Could you check a few things on this model? Use its own coordinates, in mm. Give positions to 0.01 mm unless a question says otherwise; leave off trailing zeros. Loops run counter-clockwise (first coordinate to the right, second up) from the corner with the lowest first, then second, coordinate; pieces in that order, holes last. Notation, with made-up numbers: M -20.75,69.25 L -5.75,69.25 A15 ccw -5.75,87.25 Z; hole C 38,65 d9. An arc over 180 degrees is marked long. Answer in a Markdown table with one row per item. Add a question column.
1. I'm going to push a flat-ended pin straight in: pin 1 Ø2 at (x, z) = (17.5, -1) entering from +Y. Where does the tip first touch, or does it pass through?
2. If we section it at B-B on x = 24: List the corners of the cut face in (y, z) for me.
3. If we section it at A-A on z = 0: List the corners of the cut face in (x, y) for me.
4. I need wall thicknesses on line 1 along X through (y, z) = (0, 2.15); line 2 along X through (y, z) = (0, 1.75); line 3 along Y through (x, z) = (-25, 2). Which ranges of each line are inside material? Lowest first, please. Write a range as from..to.
5. If we section it at C-C on x = -24.5: List the corners of the cut face in (y, z) for me.
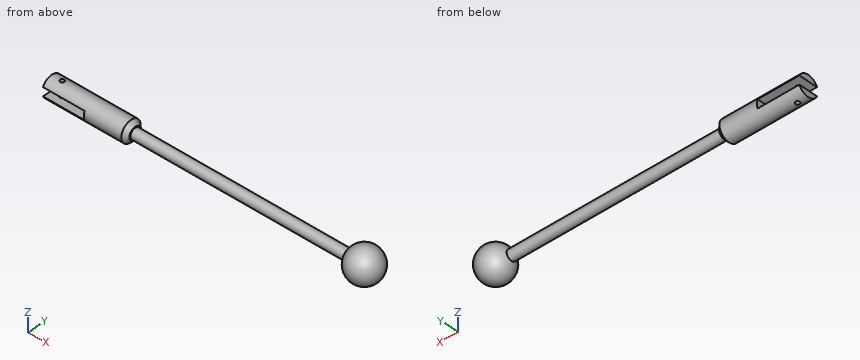
```python
from build123d import *

# Parameters (mm, degrees)
SKETCH1_W               = 75
SKETCH1_H               = 1.25
SKETCH2_R               = 2.5
BOSS_EXTRUDE1_DEPTH     = 20
SKETCH3_W               = 2.05
SKETCH3_H               = 5
CUT_EXTRUDE1_DEPTH      = 1
CUT_EXTRUDE1_DEPTH_BACK = 10
CHAMFER1_SIZE           = 1
SKETCH4_R               = 0.5
CUT_EXTRUDE2_DEPTH      = 4.525
CUT_EXTRUDE2_DEPTH_BACK = 2.475


with BuildPart() as part:
    # Sketch1 → Revolve2 (revolve)
    with BuildSketch(Plane(origin=(0, 0, 0), x_dir=(1, 0, 0), z_dir=(0, 1, 0))):
        with Locations((0, -0.625)):
            Rectangle(SKETCH1_W, SKETCH1_H)
    revolve(axis=Axis((-37.5, 0, 0), (1, 0, 0)))

    # Sketch2 → Boss-Extrude1 (add)
    with BuildSketch(Plane.ZY.offset(37.5)):
        Circle(SKETCH2_R)
    extrude(amount=-BOSS_EXTRUDE1_DEPTH)

    # Sketch3 → Cut-Extrude1 (cut, two sides)
    with BuildSketch(Plane.ZY.offset(37.5)) as cut_extrude1_sk:
        Rectangle(SKETCH3_W, SKETCH3_H)
    extrude(amount=CUT_EXTRUDE1_DEPTH, mode=Mode.SUBTRACT)
    extrude(cut_extrude1_sk.sketch, amount=-CUT_EXTRUDE1_DEPTH_BACK, mode=Mode.SUBTRACT)

    # Chamfer1
    chamfer1_edges = [part.edges().sort_by_distance(p)[0] for p in [
        (-17.5, 0, -2.5),
    ]]
    chamfer(chamfer1_edges, length=CHAMFER1_SIZE)

    # Sketch4 → Cut-Extrude2 (cut, two sides)
    with BuildSketch(Plane.XY.offset(-1.025)) as cut_extrude2_sk:
        with Locations((-35, 0)):
            Circle(SKETCH4_R)
    extrude(amount=CUT_EXTRUDE2_DEPTH, mode=Mode.SUBTRACT)
    extrude(cut_extrude2_sk.sketch, amount=-CUT_EXTRUDE2_DEPTH_BACK, mode=Mode.SUBTRACT)

    # Sketch5 one side → Revolve3 (revolve)
    with BuildSketch(Plane(origin=(37.5, 0, 0), x_dir=(0, 0, -1), z_dir=(1, 0, 0))):
        with BuildLine():
            ThreePointArc((1.25, 0), (0, 1.25), (-1.25, 0))
            Line((-1.25, 0), (1.25, 0))
        make_face()
        with BuildLine():
            Line((-4, 0), (-1.25, 0))
            ThreePointArc((-1.25, 0), (0, 1.25), (1.25, 0))
            Line((1.25, 0), (4, 0))
            ThreePointArc((4, 0), (0, 4), (-4, 0))
        make_face()
    revolve(axis=Axis((37.5, 0, 4), (0, 0, -1)))


solid = part.part
```
Results:
| question | item | result |
|---|---|---|
| 1 | pin 1 | y = 1.25 |
| 2 | outline | C 0,0 d2.5 |
| 3 | outline | M -27.5,-2.5 L -18.5,-2.5 L -17.5,-1.5 L -17.5,-1.25 L 33.7,-1.25 A4 ccw long 33.7,1.25 L -17.5,1.25 L -17.5,1.5 L -18.5,2.5 L -27.5,2.5 Z |
| 4 | line 1 | -37.5..-35.5, -34.5..-18.15, 34.13..40.87 |
| 4 | line 2 | -37.5..-35.5, -34.5..-17.75, 33.9..41.1 |
| 4 | line 3 | -1.5..1.5 |
| 5 | outline | C 0,0 d5 |
